```python
from build123d import *

# Parameters (mm, degrees)
CUT_EXTRUDE1_DEPTH = 0.75
FILLET1_R          = 0.125


with BuildPart() as part:
    # Sketch1 → Revolve1 (revolve)
    with BuildSketch(Plane(origin=(0, 0, 0), x_dir=(0, 0, -1), z_dir=(1, 0, 0))):
        with BuildLine():
            Line((0, 1.5), (-1.5, 1.5))
            ThreePointArc((-1.5, 1.5), (-1.978515811, 0.925250119), (-2.3, 0.25))
            Line((-2.3, 0.25), (-2.155662433, 0))
            Line((-2.155662433, 0), (-1, 0))
            Line((-1, 0), (-1, -12))
            Line((-1, -12), (0, -12))
            Line((0, -12), (0, 1.5))
        make_face()
    revolve(axis=Axis((0, -12, 0), (0, 1, 0)))

    # Sketch2 → Cut-Extrude1 (cut)
    with BuildSketch(Plane(origin=(0, 1.5, 0), x_dir=(1, 0, 0), z_dir=(0, 1, 0))):
        Polygon((0, 1.154700538), (-1, 0.577350269), (-1, -0.577350269), (0, -1.154700538), (1, -0.577350269), (1, 0.577350269), align=None)
    extrude(amount=-CUT_EXTRUDE1_DEPTH, mode=Mode.SUBTRACT)

    # Fillet1
    fillet1_edges = [part.edges().sort_by_distance(p)[0] for p in [
        (0.5, 1.5, -0.866025404),
        (-0.5, 1.5, -0.866025404),
        (-1, 1.5, 0),
        (-0.5, 1.5, 0.866025404),
        (0.5, 1.5, 0.866025404),
        (1, 1.5, 0),
        (0, 1.5, -1.5),
    ]]
    fillet(fillet1_edges, radius=FILLET1_R)


solid = part.part
```
Build history of the part. All positions in model axes, mm. Coordinates: 2 decimals unless noted, no trailing zeros. Order: outer loops, then holes, each group sorted by start corner. A loop starts at its lowest first (then second) coordinate and runs counter-clockwise, first axis right, second up. Notation, with made-up numbers: (21, 31.5) -> (44, 31.5) arc R14 ccw to (44, 53.5) -> close; hole circle Ø7 at (75, 16). An arc over 180 degrees is marked (long way). Answer in a Markdown table with one row per item. Add a question column.
Q1. Wall check: line 1 along Y through (x, z) = (0.5, -1.1); line 2 along X through (y, z) = (-9.5, 0.05); line 3 along Y through (x, z) = (-0.55, -0.45). Give the ranges that are in metal, low to high. Write a range as [from, to].
Q2. Mould opens along X. For faces 1 (the face through (0, 0.75, 0)), 2 (the face through (-1, -6, 0)), 3 (the face through (0, -12, 0)) say: +X half, -X half, draft (parallel to the pull), parting line (faces both ways), or undercut.
Q3. Band-saw the part on A-A, the plane y = -6. List the corners of the cut face in (x, z).
Q4. Drop flat-ended pins along their axis: pin 1 (1.5 mm diameter, centred on x = 1.5, z = 1.5, fed in from -Y); pin 2 (2 mm diameter, centred on y = -10.5, z = 1.5, fed in from -X); pin 3 (1.5 mm diameter, centred on y = -4.5, z = 0.5, fed in from -X). Give the stop position or say it passes through.
Answers follow:
| question | item | result |
|---|---|---|
| 1 | line 1 | [0, 1.5] |
| 1 | line 2 | [-1, 1] |
| 1 | line 3 | [-12, 0.75] |
| 2 | face 1 | undercut |
| 2 | face 2 | parting line |
| 2 | face 3 | draft |
| 3 | outline | circle Ø2 at (0, 0) |
| 4 | pin 1 | y = 0 |
| 4 | pin 2 | x = -0.87 |
| 4 | pin 3 | x = -1 |
